```python
from build123d import *

# Parameters (mm, degrees)
SKETCH2_R          = 7.1
CUT_EXTRUDE1_DEPTH = 63.109057311


with BuildPart() as part:
    # Sketch1 → Revolve1 (revolve)
    with BuildSketch(Plane(origin=(0, 0, 0), x_dir=(0, 0, -1), z_dir=(1, 0, 0)), mode=Mode.PRIVATE) as revolve1_sk:
        Polygon((0, 0), (41.65, 0), (41.65, -3.3), (22.523249986, -6.5), (22.523249986, -13.2), (41.65, -16.4), (41.65, -19.7), (0, -19.7), align=None)
    revolve(revolve1_sk.sketch.rotate(Axis((0, 0, 0), (0, -1, 0)), 180), axis=Axis((0, 0, 0), (0, -1, 0)))

    # Sketch2 → Cut-Extrude1 (cut, through all)
    with BuildSketch(Plane(origin=(0, 0, 0), x_dir=(1, 0, 0), z_dir=(0, 1, 0))):
        with Locations(Location((0, 0, 0), (0, 0, 270))):
            Circle(SKETCH2_R)
    extrude(amount=-CUT_EXTRUDE1_DEPTH, mode=Mode.SUBTRACT)


solid = part.part
```
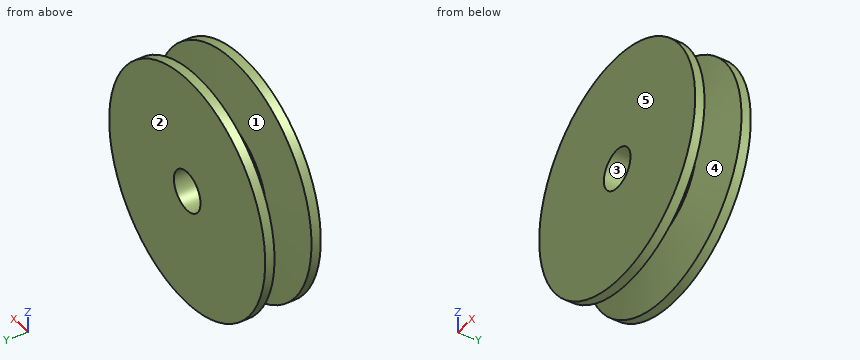
For this review, take the finished solid that the model builds, in its own axes (mm). Face numbers are marked on the shaded views. A direction names the side the tool comes from. Round coordinates to 2 decimals unless told otherwise and drop trailing zeros. Write each loop counter-clockwise with the first axis right and the second up, starting at its lowest first coordinate (ties: lowest second). Pieces come first, ordered by that corner, then holes. Notation, with made-up numbers: (29.5, -23) - (63.5, -23) arc R18 ccw to (63.5, -2) - close; hole circle Ø2 at (74, 17.25). An arc over 180 degrees is marked (long way). Answer as CSV lines item,"result". Start each with the question number.
(1) Add section B-B, the plane x = 0. State the section outline as (y, z) points, plus the area to 3 significant figures.
(2) Add section C-C, the plane y = -8.75. State the section outline as (x, z) points, plus the area to 3 significant figures.
(3) For line 1 (X direction, y = -7, z = 0); line 2 (Y direction, x = 24.5, z = 24.5); line 3 (Y direction, x = -38, z = -12.5), list the stretches that pass through material, from the lowest coordinate up.
(4) Mouldability with a two-part tool opening along X and no side actions: class the marked faces 1, 2 and 3 as +X half, -X half, draft (parallel to the pull), parting line (faces both ways), or undercut.
(5) Machinability: for the marked faces 4 and 5, which of the approach directions +Z, -Z, +X, -X, +Y, -Y give a long, thin tool a straight path to every point of the face, cutting with its end or side? Answer none if there is none.
(6) For pin 1 (22.5 mm diameter, centred on x = 0, z = 0, fed in from +Y); pin 2 (5 mm diameter, centred on y = -5.5, z = -26, fed in from +X); pin 3 (8 mm diameter, centred on y = -4.5, z = -23, fed in from +X); pin 4 (10 mm diameter, centred on x = -10, y = -2.5, fed in from -Z), all flat-tipped, find the tip position at first contact; note any pin that passes through.
(7) Add section A-A, the plane z = 0. State the section outline as (x, y) points.
From the geometry:
1,outline,"(-19.7, -41.65) - (-16.4, -41.65) - (-13.2, -22.52) - (-6.5, -22.52) - (-3.3, -41.65) - (0, -41.65) - (0, -7.1) - (-19.7, -7.1) - close; (-19.7, 7.1) - (0, 7.1) - (0, 41.65) - (-3.3, 41.65) - (-6.5, 22.52) - (-13.2, 22.52) - (-16.4, 41.65) - (-19.7, 41.65) - close"
1,area,"983 mm²"
2,outline,"circle Ø45.05 at (0, 0); hole circle Ø14.2 at (0, 0)"
2,area,"1,440 mm²"
3,line 1,"x = -22.52 to -7.1, 7.1 to 22.52"
3,line 2,"y = -19.7 to -15.23, -4.47 to 0"
3,line 3,"y = -19.7 to -16.12, -3.58 to 0"
4,face 1,"parting line"
4,face 2,"draft"
4,face 3,"undercut"
5,face 4,"none"
5,face 5,"+Z, -Z, +X, -X, -Y"
6,pin 1,"stops at y = 0"
6,pin 2,"stops at x = 33.45"
6,pin 3,"stops at x = 36.97"
6,pin 4,"stops at z = -41.35"
7,outline,"(-41.65, -19.7) - (-7.1, -19.7) - (-7.1, 0) - (-41.65, 0) - (-41.65, -3.3) - (-22.52, -6.5) - (-22.52, -13.2) - (-41.65, -16.4) - close; (7.1, -19.7) - (41.65, -19.7) - (41.65, -16.4) - (22.52, -13.2) - (22.52, -6.5) - (41.65, -3.3) - (41.65, 0) - (7.1, 0) - close"
